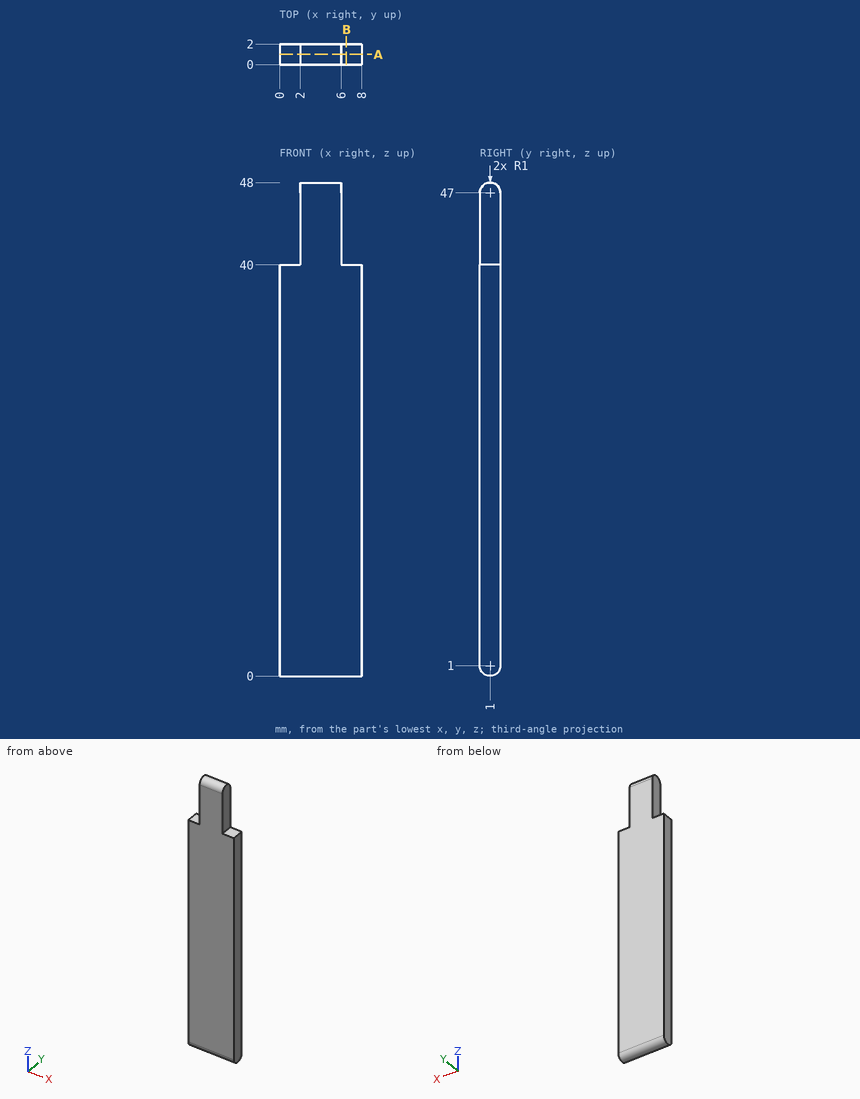
Design review of the part shown in the three views and the two pictorial views. Dimensions are in mm from the part's minimum x, y and z. Give positions to 0.01 mm unless a question says otherwise; leave off trailing zeros. Write each loop counter-clockwise with the first axis right and the second up, starting at its lowest first coordinate (ties: lowest second). Pieces come first, ordered by that corner, then holes.
(1) Clearance check with a flat-ended pin moving along its axis: pin 1 Ø0.6 at (y, z) = (1, 45.5) entering from -X. State where the tip first meets the part, or that it passes through.
Checked values:
pin 1: stops at x = 2
(2) Add section A-A (y = 1). Give the boundary of the cut face in (x, z).
Checked values:
outline: (0, 0) - (8, 0) - (8, 40) - (6, 40) - (6, 48) - (2, 48) - (2, 40) - (0, 40) - close
(3) Wall thickness on line 1 along Z through (x, y) = (3.5, 0.95); line 2 along Z through (x, y) = (7.25, 1.7): over which ranges is each line inside the solid? List them lowest first.
Checked values:
line 1: z = 0 to 48
line 2: z = 0.29 to 40
(4) Add section B-B (x = 6.5). Give the boundary of the cut face in (y, z), and give its area (3 significant figures).
Checked values:
outline: (0, 1) arc R1 ccw to (2, 1) - (2, 40) - (0, 40) - close
area: 79.6 mm2
